from build123d import *
from build123d.topology import SkipClean

# Parameters (mm, degrees)
SKETCH_1_R      = 20
SKETCH_1_R_2    = 16
EXTRUDE_1_DEPTH = 50
EXTRUDE_START   = 50
SKETCH_3_R      = 18
SKETCH_3_R_2    = 16
EXTRUDE_2_DEPTH = 10
EXTRUDE_START_2 = 60
EXTRUDE_3_DEPTH = 10


with BuildPart() as part:
    # Sketch 1 → Extrude 1 (new body)
    with BuildSketch(Plane(origin=(0, 0, 0), x_dir=(1, 0, 0), z_dir=(0, 1, 0))):
        with Locations(Location((0, 0, 0), (0, 0, 270))):
            Circle(SKETCH_1_R)
        with Locations(Location((0, 0, 0), (0, 0, 270))):
            Circle(SKETCH_1_R_2, mode=Mode.SUBTRACT)
    extrude(amount=EXTRUDE_1_DEPTH)

    # Sketch 3 → Extrude 2 (add)
    with BuildSketch(Plane(origin=(0, 0, 0), x_dir=(1, 0, 0), z_dir=(0, 1, 0)).offset(EXTRUDE_START)):
        with Locations(Location((0, 0, 0), (0, 0, 270))):
            Circle(SKETCH_3_R)
        with Locations(Location((0, 0, 0), (0, 0, 270))):
            Circle(SKETCH_3_R_2, mode=Mode.SUBTRACT)
    extrude(amount=EXTRUDE_2_DEPTH)

    # Sketch 4 → Extrude 3 (add)
    with SkipClean():  # the faces are left unmerged after this step: merging them gives an invalid solid
        with BuildSketch(Plane(origin=(0, 0, 0), x_dir=(1, 0, 0), z_dir=(0, 1, 0)).offset(EXTRUDE_START_2)):
            with BuildLine():
                Line((-17.428425058, 4.5), (-15.491933385, 4))
                ThreePointArc((-15.491933385, 4), (-11.313708499, 11.313708499), (-4, 15.491933385))
                Line((-4, 15.491933385), (-4.5, 17.428425058))
                ThreePointArc((-4.5, 17.428425058), (-12.727922061, 12.727922061), (-17.428425058, 4.5))
            make_face()
            with BuildLine():
                ThreePointArc((15.491933385, -4), (11.313708499, -11.313708499), (4, -15.491933385))
                Line((4, -15.491933385), (4.5, -17.428425058))
                ThreePointArc((4.5, -17.428425058), (12.727922061, -12.727922061), (17.428425058, -4.5))
                Line((17.428425058, -4.5), (15.491933385, -4))
            make_face()
        extrude(amount=EXTRUDE_3_DEPTH)


solid = part.part
Build history of the part. All positions in model axes, mm. A direction names the side the tool comes from. Coordinates: 2 decimals unless noted, no trailing zeros. Order: outer loops, then holes, each group sorted by start corner. A loop starts at its lowest first (then second) coordinate and runs counter-clockwise, first axis right, second up. Notation, with made-up numbers: (78, -12.75) - (125, -12.75) arc R16 ccw to (125, 5.25) - close; hole circle Ø9 at (-2, 14.5). An arc over 180 degrees is marked (long way). Write each question's results on one line, items separated by ' | '. Start each with the question number.
Item 1: Wall check: probe 1 along X at (y, z) = (35, 0); probe 2 along Z at (x, y) = (-0.5, 26.5); probe 3 along Y at (x, z) = (-9, -17.5). Give the ranges that are in metal, low to high. Write a range as [from, to].
Item 2: Tool access for faces 1 (the face through (3, 50, -18)), 2 (the face through (-16.474, 64.93, -4.254)), 3 (the face through (16.474, 64.93, 4.254)): list every direction of +Z, -Z, +X, -X, +Y, -Y with a clear straight run to the whole face (end or side of a thin tool).
Item 3: Band-saw the part on C-C on y = 31. Write the cut outline in (x, z), and give its area (3 significant figures).
Item 4: Band-saw the part on A-A on x = 0. Write the cut outline in (y, z), and give its area (3 significant figures).
Item 5: Band-saw the part on D-D on z = 14. Write the cut outline in (x, y).
Item 6: Flat gauge pins, fed straight in: pin 1 (3 mm diameter, centred on x = -13, y = 27.5, fed in from -Z); pin 2 (1.5 mm diameter, centred on y = 54.5, z = -7.5, fed in from +X); pin 3 (11 mm diameter, centred on x = 10.5, z = -3.5, fed in from +Y). Where does each tip first touch, or does it go through?
Item 7: Band-saw the part on B-B on z = 0. Write the cut outline in (x, y), and give its area (3 significant figures).
Numbers:
1) probe 1: [-20, -16], [16, 20] | probe 2: [-19.99, -15.99], [15.99, 19.99] | probe 3: [0, 50]
2) face 1: +Y | face 2: +Z, -X, +Y | face 3: -Z, +X, +Y
3) outline: circle Ø40 at (0, 0); hole circle Ø32 at (0, 0) | area: 452 mm^2
4) outline: (0, -20) - (50, -20) - (50, -18) - (60, -18) - (60, -16) - (0, -16) - close; (0, 16) - (60, 16) - (60, 18) - (50, 18) - (50, 20) - (0, 20) - close | area: 440 mm^2
5) outline: (-14.28, 0) - (-7.75, 0) - (-7.75, 60) - (-11.31, 60) - (-11.31, 50) - (-14.28, 50) - close; (7.75, 0) - (14.28, 0) - (14.28, 50) - (11.31, 50) - (11.31, 70) - (7.75, 70) - close
6) pin 1: z = -16.36 | pin 2: x = 16.69 | pin 3: y = 60
7) outline: (-20, 0) - (-16, 0) - (-16, 60) - (-18, 60) - (-18, 50) - (-20, 50) - close; (16, 0) - (20, 0) - (20, 50) - (18, 50) - (18, 60) - (16, 60) - close | area: 440 mm^2
